CAD build for the part. Positions are in the model's coordinates, mm. Round coordinates to 2 decimals unless told otherwise and drop trailing zeros. Loops run counter-clockwise (first coordinate to the right, second up) from the corner with the lowest first, then second, coordinate; pieces in that order, holes last.
```python
from build123d import *

# Parameters (mm, degrees)
SKETCH2_W           = 50
SKETCH2_H           = 150
BOSS_EXTRUDE1_DEPTH = 30
FILLET1_R           = 2
SKETCH3_W           = 99.739454276
SKETCH3_H           = 50
CUT_EXTRUDE1_DEPTH  = 0.5
SKETCH4_W           = 84.567654974
SKETCH4_H           = 50
CUT_EXTRUDE2_DEPTH  = 0.5


with BuildPart() as part:
    # Sketch2 → Boss-Extrude1 (new body)
    with BuildSketch(Plane(origin=(0, 0, 0), x_dir=(1, 0, 0), z_dir=(0, 1, 0))):
        Rectangle(SKETCH2_W, SKETCH2_H)
    extrude(amount=BOSS_EXTRUDE1_DEPTH)

    # Fillet1
    fillet1_edges = [part.edges().sort_by_distance(p)[0] for p in [
        (-25, 30, 0),
        (0, 30, 75),
        (25, 30, 0),
        (0, 0, 75),
        (-25, 0, 0),
        (0, 0, -75),
        (25, 0, 0),
        (25, 15, 75),
        (-25, 15, 75),
        (-25, 15, -75),
        (25, 15, -75),
        (0, 30, -75),
    ]]
    fillet(fillet1_edges, radius=FILLET1_R)

    # Sketch3 → Cut-Extrude1 (cut)
    with BuildSketch(Plane(origin=(0, 30, 0), x_dir=(1, 0, 0), z_dir=(0, 1, 0))):
        Rectangle(SKETCH3_W, SKETCH3_H)
    extrude(amount=-CUT_EXTRUDE1_DEPTH, mode=Mode.SUBTRACT)

    # Sketch4 → Cut-Extrude2 (cut)
    with BuildSketch(Plane.XZ):
        Rectangle(SKETCH4_W, SKETCH4_H)
    extrude(amount=-CUT_EXTRUDE2_DEPTH, mode=Mode.SUBTRACT)


solid = part.part
```
Item 1: Flat gauge pin, fed straight in: P1, Ø24.5, axis at x = -1, z = 4, coming from the -Y side. Where does the tip first touch, or does it go through?
Answers follow:
P1: stops at y = 0.5
Item 2: Cut at A-A, the plane z = -6. Give the cut face in (x, y), plus the area to 3 significant figures.
Answers follow:
outline: (-25, 2) arc R2 ccw to (-24.32, 0.5) - (24.32, 0.5) arc R2 ccw to (25, 2) - (25, 28) arc R2 ccw to (24.32, 29.5) - (-24.32, 29.5) arc R2 ccw to (-25, 28) - close
area: 1,450 mm2
Item 3: Two-plate mould, pull along Z, no slides. Class faces 1 (the flat face through (0, 29.5, 0)), 2 (the flat face through (-25, 15, 1)), 3 (the flat face through (0, 0.5, 0)), 4 (the flat face through (0, 15, -75)): released by +Z, released by -Z, zero draft, split by the parting line, or undercut.
Answers follow:
face 1: undercut
face 2: zero draft
face 3: undercut
face 4: released by -Z
Item 4: Probe line 1 (Y direction, x = -17, z = 4); line 2 (Z direction, x = -20, y = 28.5). List the from-to ranges inside material, lowest first.
Answers follow:
line 1: y = 0.5 to 29.5
line 2: z = -74.94 to 74.94
